Design review of the part shown in the three views and the two pictorial views. Dimensions are in mm from the part's minimum x, y and z. Round coordinates to 2 decimals unless told otherwise and drop trailing zeros. Loops run counter-clockwise (first coordinate to the right, second up) from the corner with the lowest first, then second, coordinate; pieces in that order, holes last. Notation, with made-up numbers: (-37.75, 37.5) -> (-3.75, 37.5) arc R16 cw to (-3.75, 65.5) -> close; hole circle Ø3 at (88, 55.25). An arc over 180 degrees is marked (long way). Return JSON: item names as keys, results as strings. Group by question number.
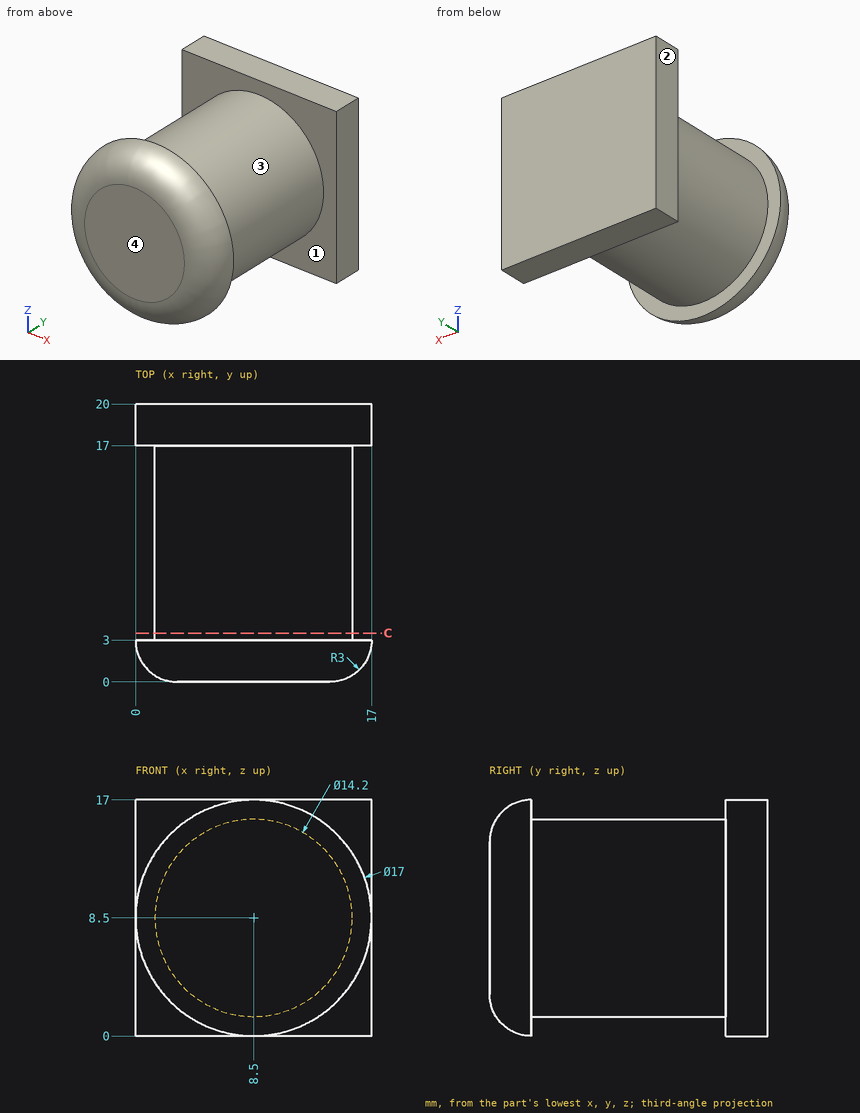
1. Wall thickness on line 1 (Y direction, x = 15, z = 2); line 2 (Y direction, x = 3, z = 10); line 3 (X direction, y = 15.5, z = 8.75): over which ranges is each line inside the solid? List them lowest first.
2. Draft analysis for pull direction Y (two halves, no side actions). For the marked faces 1, 2, 3 and 4, state which applies: pulls with the +Y half, pulls with the -Y half, needs draft (parallel to the pull), parting line crosses it, or undercut.
3. We need section C-C, the plane y = 3.5. Write out the cut boundary in (x, z).
4. For P1, Ø10, axis at y = 14.5, z = 14, coming from the -X side; P2, Ø2, axis at x = 4, y = 13, coming from the -Z side; P3, Ø10, axis at y = 9, z = 14, coming from the +X side; P4, Ø2, axis at x = 10.5, y = 9, coming from the +Z side, all flat-tipped, find the tip position at first contact; note any pin that passes through.
Check sheet entries:
{
 "1": {"line 1": "y = 17 to 20", "line 2": "y = 0.01 to 20", "line 3": "x = 1.4 to 15.6"},
 "2": {"face 1": "undercut", "face 2": "needs draft", "face 3": "undercut", "face 4": "pulls with the -Y half"},
 "3": {"outline": "circle Ø14.2 at (8.5, 8.5)"},
 "4": {"P1": "stops at x = 0", "P2": "stops at z = 2.32", "P3": "stops at x = 15.58", "P4": "stops at z = 15.53"}
}
